Can you work these out from the model? Positions are in its coordinate system, mm. A direction names the side the tool comes from. Coordinates: 2 decimals unless noted, no trailing zeros. Order: outer loops, then holes, each group sorted by start corner. A loop starts at its lowest first (then second) coordinate and runs counter-clockwise, first axis right, second up. Notation, with made-up numbers: M 38.5,43 L 80.5,43 A31 cw 80.5,81 Z; hole C 66,86.25 d11. An arc over 180 degrees is marked long. Answer as CSV lines item,"result". Start each with the question number.
1. If we mould it in two halves opening along Y, with no side actions, what happens to faces 6 (the face through (9, -8, 77)), 7 (the face through (17, -16, 41)), 8 (the face through (22, 2, 15.75))? For each: released by +Y, released by -Y, zero draft, split by the parting line, or undercut.
2. If we section it at B-B (z = 55): List the corners of the cut face in (x, y) for me, plus the area to 4 significant figures.
3. Will these pins go through, and if not, where does the flat tip stop? pin 1 (6 mm diameter, centred on x = 13.5, z = 30, fed in from -Y); pin 2 (3.5 mm diameter, centred on y = -2, z = 12.5, fed in from -X); pin 3 (3 mm diameter, centred on x = 26, z = 48.5, fed in from -Y); pin 4 (9 mm diameter, centred on x = 11.5, z = 41.5, fed in from +Y).
4. If we section it at D-D (z = 16.5): List the corners of the cut face in (x, y) for me, plus the area to 3 significant figures.
5. If we section it at A-A (x = 10): List the corners of the cut face in (y, z) for me, plus the area to 4 significant figures.
6. I need wall thicknesses on line 1 along Z through (x, y) = (15, -1); line 2 along Z through (x, y) = (13.5, -8.25); line 3 along X through (y, z) = (-7.5, 37). Which ranges of each line are inside material? Lowest first, please. Write a range as from..to.
7. If we section it at C-C (y = -7.5): List the corners of the cut face in (x, z) for me.
8. On a 3-axis mill with a long thin cutter (end or side, diameter ignored), from which of +Z, -Z, +X, -X, +Y, -Y can I reach the whole of each face in a straight line? I mean faces 1 (the face through (21, -9, 39)), 2 (the face through (7, -14, 6)), 3 (the face through (18.757, 1.726, 36.03)), 4 (the face through (15.5, -2, 15)), 5 (the face through (18, -8, 41)). Say none if no direction works.
```python
from build123d import *

# Parameters (mm, degrees)
F0_W      = 30.25
F0_H      = 80
F1_DEPTH  = 3
F2_W      = 15.5
F2_H      = 15.5
F3_DEPTH  = 3
F4_DEPTH  = 13
F6_W      = 18
F6_H      = 3
F7_DEPTH  = 3
F5_W      = 3
F5_H      = 74
F8_DEPTH  = 3
F9_W      = 15
F9_H      = 3
F10_DEPTH = 3
F11_W     = 7.5
F11_H     = 40
F12_DEPTH = 3.5
F14_DEPTH = 40


with BuildPart() as f1:
    # F0 (on Front) → F1 (new body)
    with BuildSketch(Plane.XZ):
        with Locations((15.125, 40)):
            Rectangle(F0_W, F0_H)
    extrude(amount=F1_DEPTH)

    # F2 (on face) → F3 (cut)
    with BuildSketch(Plane.XZ.offset(3)):
        with Locations((7.75, 15.5)):
            Rectangle(F2_W, F2_H)
    extrude(amount=-F3_DEPTH, mode=Mode.SUBTRACT)

    # F2 (on face) → F4 (join)
    with BuildSketch(Plane.XZ.offset(3)):
        Polygon((18, 3), (0, 3), (0, 0), (21, 0), (21, 80), (0, 80), (0, 77), (18, 77), align=None)
    extrude(amount=F4_DEPTH)

    # F6 (on face) → F7 (join)
    with BuildSketch(Plane.XY.offset(3)):
        with Locations((9, -14.5)):
            Rectangle(F6_W, F6_H)
    extrude(amount=F7_DEPTH)

    # F5 (on face) → F8 (join)
    with BuildSketch(Plane(origin=(18, 0, 0), x_dir=(0, -1, 0), z_dir=(-1, 0, 0))):
        with Locations((14.5, 40)):
            Rectangle(F5_W, F5_H)
    extrude(amount=F8_DEPTH)

    # F9 (on face) → F10 (join)
    with BuildSketch(Plane(origin=(0, 0, 77), x_dir=(1, 0, 0), z_dir=(0, 0, -1))):
        with Locations((7.5, 14.5)):
            Rectangle(F9_W, F9_H)
    extrude(amount=F10_DEPTH)

    # F11 (on face) → F12 (join)
    with BuildSketch(Plane(origin=(0, 0, 0), x_dir=(-1, 0, 0), z_dir=(0, 1, 0))):
        with Locations((-22, 35.75)):
            Rectangle(F11_W, F11_H)
    extrude(amount=F12_DEPTH)

    # F13 (on face) → F14 (cut)
    with BuildSketch(Plane.XY.offset(55.75)):
        Polygon((25.75, 0), (25.75, 3.5), (24.75, 0), align=None)
        Polygon((19.25, 0), (18.25, 3.5), (18.25, 0), align=None)
    extrude(amount=-F14_DEPTH, mode=Mode.SUBTRACT)


solid = f1.part
```
Solved:
1,face 6,"undercut"
1,face 7,"released by -Y"
1,face 8,"zero draft"
2,outline,"M 0,-3 L 18,-3 L 18,-13 L 15,-13 L 15,-16 L 21,-16 L 21,-3 L 30.25,-3 L 30.25,0 L 24.75,0 L 25.75,3.5 L 18.25,3.5 L 19.25,0 L 0,0 Z"
2,area,"161.5 mm²"
3,pin 1,"y = -16"
3,pin 2,"x = 15.5"
3,pin 3,"y = -3"
3,pin 4,"y = 0"
4,outline,"M 15,-16 L 21,-16 L 21,-3 L 30.25,-3 L 30.25,0 L 24.75,0 L 25.75,3.5 L 18.25,3.5 L 19.25,0 L 15.5,0 L 15.5,-3 L 18,-3 L 18,-13 L 15,-13 Z"
4,area,"115 mm²"
5,outline,"M -16,0 L 0,0 L 0,7.75 L -3,7.75 L -3,3 L -13,3 L -13,6 L -16,6 Z; M -16,74 L -13,74 L -13,77 L -3,77 L -3,23.25 L 0,23.25 L 0,80 L -16,80 Z"
5,area,"289.5 mm²"
6,line 1,"0..7.75, 23.25..80"
6,line 2,"0..3, 77..80"
6,line 3,"18..21"
7,outline,"M 0,0 L 21,0 L 21,80 L 0,80 L 0,77 L 18,77 L 18,3 L 0,3 Z"
8,face 1,"+Z, -Z, +X, -Y"
8,face 2,"-X, -Y"
8,face 3,"+Z, -Z, -X"
8,face 4,"-X, +Y"
8,face 5,"-X"
